Here's the drawing with two shaded views (mm, measured from the low corner). I have some questions. A direction names the side the tool comes from. Coordinates: 2 decimals unless noted, no trailing zeros. Write each loop counter-clockwise with the first axis right and the second up, starting at its lowest first coordinate (ties: lowest second). Pieces come first, ordered by that corner, then holes. Notation, with made-up numbers: M 81.25,-4.75 L 135.25,-4.75 A30 cw 135.25,20.25 Z; hole C 87,55.25 d5. An arc over 180 degrees is marked long. Use one line per item in the form item = value. Start each with the question number.
1. On a 3-axis mill with a long thin cutter (end or side, diameter ignored), from which of +Z, -Z, +X, -X, +Y, -Y can I reach the whole of each face in a straight line? I mean the marked faces 1 and 2. Say none if no direction works.
2. I want a section at A-A, the plane x = 10. List the corners of the cut face in (y, z) for me.
3. Please list where these lines run through material, in increasing order: line 1 along Y through (x, z) = (16, 5.5); line 2 along X through (y, z) = (9, 6.75); line 3 along X through (y, z) = (87.5, 10.25). Write a range as [from, to].
4. I want a section at B-B, the plane z = 5.25. List the corners of the cut face in (x, y) for me, plus the area to 3 significant figures.
5. I'm going to push flat-ended pins straight in: pin 1 Ø5 at (y, z) = (88, 13.5) entering from -X; pin 2 Ø2 at (x, y) = (10.5, 54) entering from -Z; pin 3 Ø1 at (x, y) = (3, 73) entering from -Z. Where does each tip first touch, or does it pass through?
6. I want a section at C-C, the plane y = 79. List the corners of the cut face in (x, z) for me.
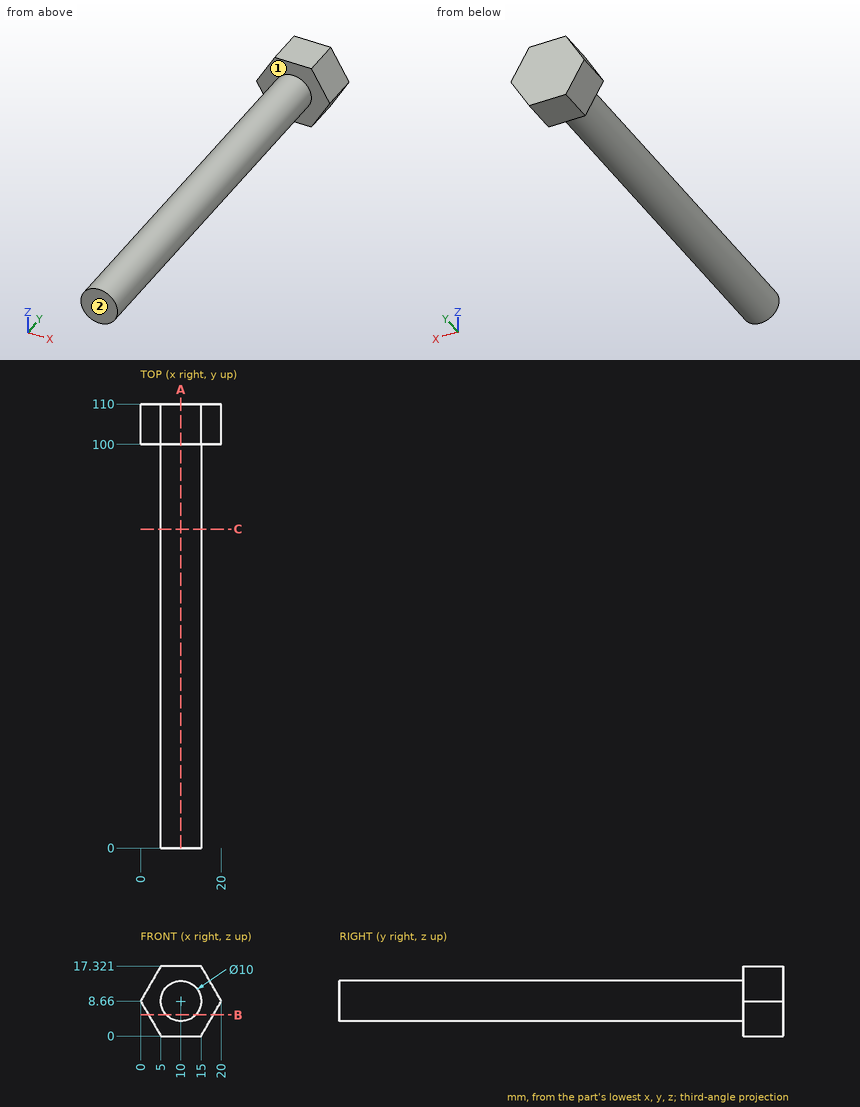
Answer list:
q1.face_1 = -Y
q1.face_2 = +Z, -Z, +X, -X, -Y
q2.outline = M 0,3.66 L 100,3.66 L 100,0 L 110,0 L 110,17.32 L 100,17.32 L 100,13.66 L 0,13.66 Z
q3.line_1 = [100, 110]
q3.line_2 = [5.38, 14.62]
q3.line_3 = [5.26, 14.74]
q4.outline = M 1.97,100 L 6.34,100 L 6.34,0 L 13.66,0 L 13.66,100 L 18.03,100 L 18.03,110 L 1.97,110 Z
q4.area = 892 mm²
q5.pin_1 = 5.58
q5.pin_2 = 3.66
q5.pin_3 = through
q6.outline = C 10,8.66 d10
